from build123d import *

# Parameters (mm, degrees)
CROQUIS1_R              = 1.65
SALIENTE_EXTRUIR1_DEPTH = 2
SALIENTE_EXTRUIR2_DEPTH = 2
REDONDEO1_R             = 1
REDONDEO2_R             = 2
CROQUIS3_R              = 2
CORTAR_EXTRUIR1_DEPTH   = 60.39696962


with BuildPart() as part:
    # Croquis1 → Saliente-Extruir1 (new body)
    with BuildSketch(Plane(origin=(0, 0, 0), x_dir=(0, 0, -1), z_dir=(1, 0, 0))):
        with BuildLine():
            Line((0, 18.8), (-20.8, 18.8))
            Line((-20.8, 18.8), (-20.8, -18.8))
            Line((-20.8, -18.8), (0, -18.8))
            ThreePointArc((0, -18.8), (18.8, 0), (0, 18.8))
        make_face()
        with Locations((13.423393759, 7.75)):
            Circle(CROQUIS1_R, mode=Mode.SUBTRACT)
        with Locations((13.423393759, -7.75)):
            Circle(CROQUIS1_R, mode=Mode.SUBTRACT)
        with Locations((0, -15.5)):
            Circle(CROQUIS1_R, mode=Mode.SUBTRACT)
        with Locations((-13.423393759, -7.75)):
            Circle(CROQUIS1_R, mode=Mode.SUBTRACT)
        with Locations((-13.423393759, 7.75)):
            Circle(CROQUIS1_R, mode=Mode.SUBTRACT)
        with Locations((0, 15.5)):
            Circle(CROQUIS1_R, mode=Mode.SUBTRACT)
        with BuildLine():
            Line((-7, 6.6), (7, 6.6))
            ThreePointArc((7, 6.6), (13.6, 0), (7, -6.6))
            Line((7, -6.6), (-7, -6.6))
            ThreePointArc((-7, -6.6), (-13.6, 0), (-7, 6.6))
        make_face(mode=Mode.SUBTRACT)
    extrude(amount=SALIENTE_EXTRUIR1_DEPTH)

    # Croquis2 → Saliente-Extruir2 (add)
    with BuildSketch(Plane.XY.offset(20.8)):
        Polygon((2, 18.8), (-38, 18.8), (-38, -18.150603338), (2, -18.8), align=None)
    extrude(amount=SALIENTE_EXTRUIR2_DEPTH)

    # Redondeo1
    redondeo1_edges = [part.edges().sort_by_distance(p)[0] for p in [
        (2, 0, 22.8),
    ]]
    fillet(redondeo1_edges, radius=REDONDEO1_R)

    # Redondeo2
    redondeo2_edges = [part.edges().sort_by_distance(p)[0] for p in [
        (-38, 18.8, 21.8),
        (-38, -18.150603338, 21.8),
    ]]
    fillet(redondeo2_edges, radius=REDONDEO2_R)

    # Croquis3 → Cortar-Extruir1 (cut, through all)
    with BuildSketch(Plane.XY.offset(22.8)):
        with Locations((-7, 14.8)):
            Circle(CROQUIS3_R)
        with Locations(Location((-7, -14.783765083, 0), (0, 0, 180))):
            Circle(CROQUIS3_R)
        with Locations((-30.5, 14.8)):
            Circle(CROQUIS3_R)
        with Locations((-30.5, -14.783765083)):
            Circle(CROQUIS3_R)
    extrude(amount=-CORTAR_EXTRUIR1_DEPTH, mode=Mode.SUBTRACT)


solid = part.part
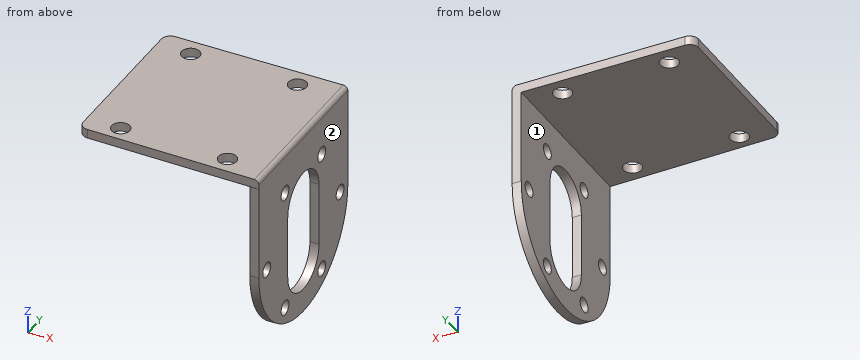
Can you work these out from the model? Positions are in its coordinate system, mm. Face numbers are marked on the shaded views. A direction names the side the tool comes from. Round coordinates to 2 decimals unless told otherwise and drop trailing zeros. Write each loop counter-clockwise with the first axis right and the second up, starting at its lowest first coordinate (ties: lowest second). Pieces come first, ordered by that corner, then holes. Notation, with made-up numbers: (4.5, 6) - (54.5, 6) arc R7 cw to (54.5, 14) - close; hole circle Ø2 at (-25, 88.5). An arc over 180 degrees is marked (long way). Write each question's results on one line, items separated by ' | '. Start each with the question number.
1) Suppose I cut it at C-C (x = -30.5). List the corners of the cut face in (y, z) for me, and give its area (3 significant figures).
2) Which directions (+Z, -Z, +X, -X, +Y, -Y) give clear straight access to the entire face, cutting with the end or side of a thin tool? Please do the marked faces 1 and 2.
3) Suppose I cut it at B-B (z = 3.5). List the corners of the cut face in (x, y) for me.
4) Please list where these lines run through material, in increasing order: line 1 (Y direction, x = -30.5, z = 22.25); line 2 (Z direction, x = -20, y = -17); line 3 (X direction, y = -7, z = -5).
5) Suppose I cut it at D-D (y = 14.8). List the corners of the cut face in (x, z) for me, and give its area (3 significant figures).
6) For pin 1 Ø4.5 at (y, z) = (7.75, 13.42) entering from -X; pin 2 Ø19 at (x, y) = (-25.5, 4.5) entering from -Z, each with a flat end and sliding along its axis, tell me the tip position at first contact or that it passes through.
7) Suppose I cut it at A-A (y = 0). List the corners of the cut face in (x, z) for me, and give its area (3 significant figures).
Here are the results:
1) outline: (-18.27, 20.8) - (-16.78, 20.8) - (-16.78, 22.8) - (-18.27, 22.8) - close; (-12.78, 20.8) - (12.8, 20.8) - (12.8, 22.8) - (-12.78, 22.8) - close; (16.8, 20.8) - (18.8, 20.8) - (18.8, 22.8) - (16.8, 22.8) - close | area: 58.1 mm2
2) face 1: -Z, -X, +Y, -Y | face 2: +Z, -Z, +X, +Y, -Y
3) outline: (0, -18.8) - (2, -18.8) - (2, -6.6) - (0, -6.6) - close; (0, 6.6) - (2, 6.6) - (2, 18.8) - (0, 18.8) - close
4) line 1: y = -18.27 to -16.78, -12.78 to 12.8, 16.8 to 18.8 | line 2: z = 20.8 to 22.8 | line 3: x = 0 to 2
5) outline: (-38, 20.8) - (-32.5, 20.8) - (-32.5, 22.8) - (-38, 22.8) - close; (-28.5, 20.8) - (-9, 20.8) - (-9, 22.8) - (-28.5, 22.8) - close; (-5, 20.8) - (0, 20.8) - (0, 1.49) - (2, 1.49) - (2, 21.8) arc R1 ccw to (1, 22.8) - (-5, 22.8) - close; (0, -11.59) - (2, -11.59) - (2, -1.49) - (0, -1.49) - close | area: 123 mm2
6) pin 1: stops at x = 0 | pin 2: stops at z = 20.8
7) outline: (-38, 20.8) - (0, 20.8) - (0, 13.6) - (2, 13.6) - (2, 21.8) arc R1 ccw to (1, 22.8) - (-38, 22.8) - close; (0, -18.8) - (2, -18.8) - (2, -13.6) - (0, -13.6) - close | area: 105 mm2
